Source: CAD feature listing. Evaluate the final solid. Frame: model axes, mm. A direction names the side the tool comes from. Coordinates: 2 decimals unless noted, no trailing zeros. Loops run counter-clockwise (first coordinate to the right, second up) from the corner with the lowest first, then second, coordinate; pieces in that order, holes last. Notation, with made-up numbers: (50.5, -4) -> (58.5, -4) arc R22 cw to (58.5, 32) -> close; hole circle Ø4 at (44, 33.5). An arc over 180 degrees is marked (long way). One line per question, with ' | ' between items. Start each with the question number.
Autodesk Inventor part; units mm, degrees
ref_plane "YZ Plane" through (0, 0, 0) normal (1, 0, 0) x (0, 1, 0)
ref_plane "XZ Plane" through (0, 0, 0) normal (0, 1, 0) x (-1, 0, 0)
ref_plane "XY Plane" through (0, 0, 0) normal (0, 0, 1) x (1, 0, 0)
sketch "Sketch1" plane through (0, 0, 0) normal (0, 1, 0) x (-1, 0, 0)
  line L0 (0, 0) -> (-100, 0)
  line L1 (-100, 0) -> (-100, -24.25)
  line L2 (-100, -24.25) -> (-86, -24.25)
  arc A0 (-86, -50.25) -> (-86, -24.25) centre (-86, -37.25) ccw
  line L3 (-86, -50.25) -> (-100, -50.25)
  line L4 (-100, -50.25) -> (-100, -74.5)
  line L5 (-100, -74.5) -> (0, -74.5)
  line L6 (0, -74.5) -> (0, -50.25)
  line L7 (0, -50.25) -> (-14, -50.25)
  arc A1 (-14, -24.25) -> (-14, -50.25) centre (-14, -37.25) ccw
  line L8 (-14, -24.25) -> (0, -24.25)
  line L9 (0, -24.25) -> (0, 0)
  circle A2 centre (-14, -62.25) radius 2.25
  circle A3 centre (-14, -12.25) radius 2.25
  circle A4 centre (-86, -62.25) radius 2.25
  circle A5 centre (-86, -12.25) radius 2.25
  dimension "d0" = 13
  dimension "d1" = 50
  dimension "d2" = 4.5
  dimension "d3" = 25
  dimension "d5" = 12.25
  dimension "d6" = 100
  dimension "d10" = 14
extrude "Extrusion1" add sketch "Sketch1" along normal blind 6.5
sketch "Sketch3" plane through (0, 6.5, 0) normal (0, 1, 0) x (1, 0, 0)
  line L0 (100, 74.5) -> (0, 74.5)
  line L1 (22.75, 74.5) -> (27.25, 74.5)
  line L2 (27.25, 58.2) -> (22.75, 58.2)
  line L3 (29.75, 69.5) -> (29.75, 62.2)
  line L4 (20.25, 62.2) -> (20.25, 69.5)
  line L5 (27.25, 74.5) -> (27.25, 69.5)
  line L6 (27.25, 62.2) -> (27.25, 58.2)
  line L7 (22.75, 58.2) -> (22.75, 62.2)
  line L8 (22.75, 69.5) -> (22.75, 74.5)
  line L9 (20.25, 69.5) -> (22.75, 69.5)
  line L10 (27.25, 69.5) -> (29.75, 69.5)
  line L11 (29.75, 62.2) -> (27.25, 62.2)
  line L12 (22.75, 62.2) -> (20.25, 62.2)
  line L13 (72.75, 74.5) -> (77.25, 74.5)
  line L14 (77.25, 58.2) -> (72.75, 58.2)
  line L15 (79.75, 69.5) -> (79.75, 62.2)
  line L16 (70.25, 62.2) -> (70.25, 69.5)
  line L17 (77.25, 74.5) -> (77.25, 69.5)
  line L18 (77.25, 62.2) -> (77.25, 58.2)
  line L19 (72.75, 58.2) -> (72.75, 62.2)
  line L20 (72.75, 69.5) -> (72.75, 74.5)
  line L21 (70.25, 69.5) -> (72.75, 69.5)
  line L22 (77.25, 69.5) -> (79.75, 69.5)
  line L23 (79.75, 62.2) -> (77.25, 62.2)
  line L24 (72.75, 62.2) -> (70.25, 62.2)
  line L25 (29.75, 65.85) -> (70.25, 65.85) construction
  point P0 (25, 58.2)
  point P1 (75, 58.2)
  point P2 (50, 65.85)
  point P3 (50, 74.5)
  dimension "d15" = 4.5
  dimension "d16" = 2.5
  dimension "d17" = 4
  dimension "d18" = 5
  dimension "d19" = 7.3
  dimension "d20" = 4.5
  dimension "d21" = 2.5
  dimension "d22" = 4
  dimension "d23" = 5
  dimension "d24" = 7.3
  dimension "d25" = 50
extrude "Extrusion2" cut sketch "Sketch3" against normal through all
sketch "Sketch4" plane through (0, 6.5, 0) normal (0, 1, 0) x (1, 0, 0)
  line L0 (22.75, 74.5) -> (0, 74.5)
  line L1 (100, 74.5) -> (77.25, 74.5)
  line L2 (77.25, 58.2) -> (72.75, 58.2)
  line L3 (72.75, 74.5) -> (27.25, 74.5)
  line L4 (27.25, 58.2) -> (22.75, 58.2)
  line L5 (9.5, 74.5) -> (17.5, 74.5)
  line L6 (17.5, 74.5) -> (17.5, 95.7)
  line L7 (15.5, 97.7) -> (11.5, 97.7)
  line L8 (9.5, 95.7) -> (9.5, 74.5)
  line L9 (32.5, 74.5) -> (40.5, 74.5)
  line L10 (40.5, 74.5) -> (40.5, 95.7)
  line L11 (38.5, 97.7) -> (34.5, 97.7)
  line L12 (32.5, 95.7) -> (32.5, 74.5)
  line L13 (59.5, 74.5) -> (67.5, 74.5)
  line L14 (67.5, 74.5) -> (67.5, 95.7)
  line L15 (65.5, 97.7) -> (61.5, 97.7)
  line L16 (59.5, 95.7) -> (59.5, 74.5)
  line L17 (82.5, 74.5) -> (90.5, 74.5)
  line L18 (90.5, 74.5) -> (90.5, 95.7)
  line L19 (88.5, 97.7) -> (84.5, 97.7)
  line L20 (82.5, 95.7) -> (82.5, 74.5)
  arc A0 (11.5, 97.7) -> (9.5, 95.7) centre (11.5, 95.7) ccw
  arc A1 (17.5, 95.7) -> (15.5, 97.7) centre (15.5, 95.7) ccw
  arc A2 (34.5, 97.7) -> (32.5, 95.7) centre (34.5, 95.7) ccw
  arc A3 (40.5, 95.7) -> (38.5, 97.7) centre (38.5, 95.7) ccw
  arc A4 (61.5, 97.7) -> (59.5, 95.7) centre (61.5, 95.7) ccw
  arc A5 (67.5, 95.7) -> (65.5, 97.7) centre (65.5, 95.7) ccw
  arc A6 (84.5, 97.7) -> (82.5, 95.7) centre (84.5, 95.7) ccw
  arc A7 (90.5, 95.7) -> (88.5, 97.7) centre (88.5, 95.7) ccw
  point P0 (25, 58.2)
  point P1 (75, 58.2)
  dimension "d28" = 2
  dimension "d29" = 23.2
  dimension "d30" = 8
  dimension "d31" = 8
  dimension "d32" = 8
  dimension "d33" = 8
  dimension "d34" = 15
  dimension "d35" = 15
  dimension "d36" = 7.5
  dimension "d37" = 7.5
extrude "Extrusion3" add sketch "Sketch4" against normal blind 6.5
chamfer "Chamfer1" distance 4 angle 45 2 edges at (100, 3.25, 0) (0, 3.25, 0)
chamfer "Chamfer2" distance 2 angle 45 4 edges at (100, 3.25, -24.25) (100, 3.25, -50.25) (0, 3.25, -50.25) (0, 3.25, -24.25)
sketch "Sketch5" plane through (0, 6.5, 0) normal (0, 1, 0) x (1, 0, 0)
  line L0 (4, 0) -> (96, 0)
  line L1 (34.25, 16) -> (40.75, 16)
  line L2 (40.75, 16) -> (40.75, 8)
  line L3 (40.75, 8) -> (34.25, 8)
  line L4 (34.25, 8) -> (34.25, 16)
  line L5 (59.25, 16) -> (65.75, 16)
  line L6 (65.75, 16) -> (65.75, 8)
  line L7 (65.75, 8) -> (59.25, 8)
  line L8 (59.25, 8) -> (59.25, 16)
  circle A0 centre (37.5, 36) radius 2.25
  circle A1 centre (62.5, 36) radius 2.25
  line L9 (37.5, 36) -> (62.5, 36) construction
  point P0 (0, 0)
  point P1 (37.5, 16)
  point P2 (62.5, 16)
  point P3 (50, 36)
  point P4 (50, 0)
  dimension "d46" = 4.5
  dimension "d47" = 6.5
  dimension "d48" = 8
  dimension "d49" = 25
  dimension "d50" = 8
  dimension "d51" = 20
extrude "Extrusion4" cut sketch "Sketch5" against normal through all
sketch "Sketch6" plane through (0, 6.5, 0) normal (0, 1, 0) x (1, 0, 0)
  line L0 (59.5, 74.5) -> (40.5, 74.5)
  line L1 (46.75, 40.5) -> (53.25, 40.5)
  line L2 (53.25, 40.5) -> (53.25, 32.5)
  line L3 (53.25, 32.5) -> (46.75, 32.5)
  line L4 (46.75, 32.5) -> (46.75, 40.5)
  circle A0 centre (50, 48) radius 2.25
  point P0 (0, 0)
  point P1 (50, 74.5)
  point P2 (50, 40.5)
  dimension "d54" = 6.5
  dimension "d55" = 8
  dimension "d56" = 4.5
  dimension "d57" = 7.5
  dimension "d58" = 34
extrude "Extrusion5" cut sketch "Sketch6" against normal through all
sketch "Sketch7" plane through (0, 0, 0) normal (0, -1, 0) x (1, 0, 0)
  line L0 (59.5, -74.5) -> (40.5, -74.5)
  line L1 (45.75, -74.5) -> (54.25, -74.5)
  line L2 (54.25, -74.5) -> (54.25, -68.5)
  line L3 (54.25, -68.5) -> (45.75, -68.5)
  line L4 (45.75, -68.5) -> (45.75, -74.5)
  point P0 (0, 0)
  point P1 (50, -68.5)
  point P2 (50, -74.5)
  dimension "d61" = 8.5
  dimension "d62" = 6
extrude "Extrusion6" cut sketch "Sketch7" against normal through all
chamfer "Chamfer3" distance 1.5 angle 45 2 edges at (54.25, 3.25, -68.5) (45.75, 3.25, -68.5)
equation "\"d3\" = 0.5 * d1"
equation "\"d31\" = d30"
equation "\"d32\" = d31"
equation "\"d33\" = d32"
properties part number "x_carryage_extruder_mount" material "Plywood, Finish"
(1) Cut plane A-A, the plane z = -12.25. Return the cut outline in (x, y), and give its area (3 significant figures).
(2) Cut plane D-D, the plane z = -48. Return the cut outline in (x, y).
(3) Contact query for flat-ended pins moving along their axis: pin 1 Ø2 at (x, y) = (29, 3.5) entering from -Z; pin 2 Ø2 at (y, z) = (2.5, -83.5) entering from -X. Output: stop coordinate, or through.
(4) Cut plane B-B, the plane z = -82. Return the cut outline in (x, y), and give its area (3 significant figures).
(5) Access query for faces 1 (the flat face through (95, 3, -74.5)), 2 (the flat face through (32.5, 3, -85)), 3 (the flat face through (53.25, 3, -37)), 4 (the flat face through (8, 3, -50.25)), 5 (the flat face through (98, 3, -2)). Directions: +Z, -Z, +X, -X, +Y, -Y. A direction counts if a zero-diameter tool reaches every point of the face in a straight line with its end or side. Return the directions, or none.
(6) Ray query, L1, parallel to X at y = 3.5, z = -83; L2, parallel to Z at x = 86, y = 3.5. Return the intervals inside material, ascending.
(7) Cut plane C-C, the plane x = 24. Return the cut outline in (y, z), and give its area (3 significant figures).
(8) Draft query along Z for faces 6 (the cylindrical face through (83.854, 3.204, -12.926)), 7 (the flat face through (8, 3, -24.25)), 8 (the flat face through (27.25, 3, -60)), 9 (the flat face through (70, 3, -74.5)). Return one class per face: pulls with the +Z half, pulls with the -Z half, needs draft (parallel to the pull), parting line crosses it, or undercut.
Here are the results:
1) outline: (0, 0) -> (11.75, 0) -> (11.75, 6.5) -> (0, 6.5) -> close; (16.25, 0) -> (34.25, 0) -> (34.25, 6.5) -> (16.25, 6.5) -> close; (40.75, 0) -> (59.25, 0) -> (59.25, 6.5) -> (40.75, 6.5) -> close; (65.75, 0) -> (83.75, 0) -> (83.75, 6.5) -> (65.75, 6.5) -> close; (88.25, 0) -> (100, 0) -> (100, 6.5) -> (88.25, 6.5) -> close | area: 507 mm2
2) outline: (21.31, 0) -> (47.75, 0) -> (47.75, 6.5) -> (21.31, 6.5) -> close; (52.25, 0) -> (78.69, 0) -> (78.69, 6.5) -> (52.25, 6.5) -> close
3) pin 1: stops at z = -74.5 | pin 2: stops at x = 9.5
4) outline: (9.5, 0) -> (17.5, 0) -> (17.5, 6.5) -> (9.5, 6.5) -> close; (32.5, 0) -> (40.5, 0) -> (40.5, 6.5) -> (32.5, 6.5) -> close; (59.5, 0) -> (67.5, 0) -> (67.5, 6.5) -> (59.5, 6.5) -> close; (82.5, 0) -> (90.5, 0) -> (90.5, 6.5) -> (82.5, 6.5) -> close | area: 208 mm2
5) face 1: -Z, +X, +Y, -Y | face 2: -Z, +Y, -Y | face 3: +Y, -Y | face 4: -X, +Y, -Y | face 5: +Z, +X, +Y, -Y
6) L1: x = 9.5 to 17.5, 32.5 to 40.5, 59.5 to 67.5, 82.5 to 90.5 | L2: z = -97.7 to -64.5, -60 to -50.25, -24.25 to -14.5, -10 to 0
7) outline: (0, -58.2) -> (6.5, -58.2) -> (6.5, -45.56) -> (0, -45.56) -> close; (0, -28.94) -> (6.5, -28.94) -> (6.5, 0) -> (0, 0) -> close | area: 270 mm2
8) face 6: undercut | face 7: undercut | face 8: needs draft | face 9: pulls with the -Z half
